The model under review builds one solid part; all positions refer to its coordinate system, in mm. A direction names the side the tool comes from. Give positions to 0.01 mm unless a question says otherwise; leave off trailing zeros. Loops run counter-clockwise (first coordinate to the right, second up) from the corner with the lowest first, then second, coordinate; pieces in that order, holes last. Notation, with made-up numbers: (-30, 32) -> (17, 32) arc R12 cw to (17, 45) -> close; hole circle Ø1 at (-13.5, -31.5). An arc over 180 degrees is marked (long way). Write each question's results on one line, items separated by ' | '. Start each with the question number.
Q1. Mouldability with a two-part tool opening along X and no side actions: class faces 1 (the face through (12, 12.7, 1)), 2 (the face through (12, 20.2, 1)), 3 (the face through (29, 0, 1)) as released by +X, released by -X, zero draft, split by the parting line, or undercut.
Q2. Insertion check: pin 1 Ø10 at (y, z) = (3.5, 8.5) entering from +X; pin 2 Ø1.4 at (x, y) = (23, 14.5) entering from +Z; pin 3 Ø12 at (x, z) = (22.5, 12.5) entering from +Y (3 decimals); pin 4 Ø10 at (x, y) = (8.5, -14.5) entering from +Z. Each pin has a flat end and moves straight along its axis. Give the tip position at first contact, or say it passes through.
Q3. We need section A-A (z = 20.5). Write out the cut boundary in (x, y) (3 decimals).
Q4. We need section D-D (x = 24). Write out the cut boundary in (y, z) (3 decimals), plus the area to 3 significant figures.
Q5. Machinability: for faces 4 (the face through (21.5, 0, 1)), 5 (the face through (12, -20.2, 1)), 6 (the face through (23.49, 12.88, 11.37)), which of the approach directions +Z, -Z, +X, -X, +Y, -Y give a long, thin tool a straight path to every point of the face, cutting with its end or side? Answer none if there is none.
Q6. We need section B-B (y = 5.5). Write out the cut boundary in (x, z), plus the area to 3 significant figures.
Q7. Wall thickness on L1, parallel to Y at x = 24, z = 11.75 (3 decimals); L2, parallel to Z at x = 2, y = -7; L3, parallel to Y at x = -0.5, z = 11.5: over which ranges is each line inside the solid? List them lowest first. Write a range as [from, to].
Q8. We need section C-C (x = 18.5). Write out the cut boundary in (y, z), plus the area to 3 significant figures.
from build123d import *

# Parameters (mm, degrees)
SKETCH1_W           = 34
SKETCH1_H           = 40.4
SKETCH1_W_2         = 19
SKETCH1_H_2         = 25.4
BOSS_EXTRUDE1_DEPTH = 2
SKETCH1_3_R         = 2.375
BOSS_EXTRUDE2_DEPTH = 21
CUT_EXTRUDE1_START  = 21
SKETCH1_4_R         = 1.25
CUT_EXTRUDE1_DEPTH  = 15
SKETCH1_6_R         = 2.375
BOSS_EXTRUDE3_DEPTH = 24.5
CUT_EXTRUDE2_START  = 24.5
SKETCH1_8_R         = 1.25
CUT_EXTRUDE2_DEPTH  = 18.5


with BuildPart() as part:
    # Sketch1 → Boss-Extrude1 (new body)
    with BuildSketch(Plane.XY):
        with Locations((12, 0)):
            Rectangle(SKETCH1_W, SKETCH1_H)
        with Locations((12, 0)):
            Rectangle(SKETCH1_W_2, SKETCH1_H_2, mode=Mode.SUBTRACT)
    extrude(amount=BOSS_EXTRUDE1_DEPTH)

    # Sketch1<3> → Boss-Extrude2 (add)
    with BuildSketch(Plane.XY):
        with Locations((0, 15.2)):
            Circle(SKETCH1_3_R)
        with Locations((24, 15.2)):
            Circle(SKETCH1_3_R)
    extrude(amount=BOSS_EXTRUDE2_DEPTH)

    # Sketch1<4> → Cut-Extrude1 (cut)
    with BuildSketch(Plane.XY.offset(CUT_EXTRUDE1_START)):
        with Locations((0, 15.2)):
            Circle(SKETCH1_4_R)
        with Locations((24, 15.2)):
            Circle(SKETCH1_4_R)
        with Locations((24, -15.2)):
            Circle(SKETCH1_4_R)
        with Locations((0, -15.2)):
            Circle(SKETCH1_4_R)
    extrude(amount=-CUT_EXTRUDE1_DEPTH, mode=Mode.SUBTRACT)

    # Sketch1<6> → Boss-Extrude3 (add)
    with BuildSketch(Plane.XY):
        with Locations((24, -15.2)):
            Circle(SKETCH1_6_R)
        with Locations((0, -15.2)):
            Circle(SKETCH1_6_R)
    extrude(amount=BOSS_EXTRUDE3_DEPTH)

    # Sketch1<8> → Cut-Extrude2 (cut)
    with BuildSketch(Plane.XY.offset(CUT_EXTRUDE2_START)):
        with Locations((0, -15.2)):
            Circle(SKETCH1_8_R)
        with Locations((24, -15.2)):
            Circle(SKETCH1_8_R)
    extrude(amount=-CUT_EXTRUDE2_DEPTH, mode=Mode.SUBTRACT)


solid = part.part
Output:
1) face 1: undercut | face 2: zero draft | face 3: released by +X
2) pin 1: through | pin 2: z = 21 | pin 3: y = 17.575 | pin 4: z = 2
3) outline: circle Ø4.75 at (0, -15.2); circle Ø4.75 at (0, 15.2); circle Ø4.75 at (24, -15.2); circle Ø4.75 at (24, 15.2); hole circle Ø2.5 at (0, -15.2); hole circle Ø2.5 at (0, 15.2); hole circle Ø2.5 at (24, -15.2); hole circle Ø2.5 at (24, 15.2)
4) outline: (-20.2, 0) -> (20.2, 0) -> (20.2, 2) -> (17.575, 2) -> (17.575, 21) -> (16.45, 21) -> (16.45, 6) -> (13.95, 6) -> (13.95, 21) -> (12.825, 21) -> (12.825, 2) -> (-12.825, 2) -> (-12.825, 24.5) -> (-13.95, 24.5) -> (-13.95, 6) -> (-16.45, 6) -> (-16.45, 24.5) -> (-17.575, 24.5) -> (-17.575, 2) -> (-20.2, 2) -> close | area: 194 mm2
5) face 4: +Z, -Z | face 5: +Z, -Z, +X, -X, -Y | face 6: +Z
6) outline: (-5, 0) -> (2.5, 0) -> (2.5, 2) -> (-5, 2) -> close; (21.5, 0) -> (29, 0) -> (29, 2) -> (21.5, 2) -> close | area: 30.0 mm2
7) L1: [-17.575, -16.45], [-13.95, -12.825], [12.825, 13.95], [16.45, 17.575] | L2: [0, 2] | L3: [-17.52, -16.35], [-14.05, -12.88], [12.88, 14.05], [16.35, 17.52]
8) outline: (-20.2, 0) -> (-12.7, 0) -> (-12.7, 2) -> (-20.2, 2) -> close; (12.7, 0) -> (20.2, 0) -> (20.2, 2) -> (12.7, 2) -> close | area: 30.0 mm2
